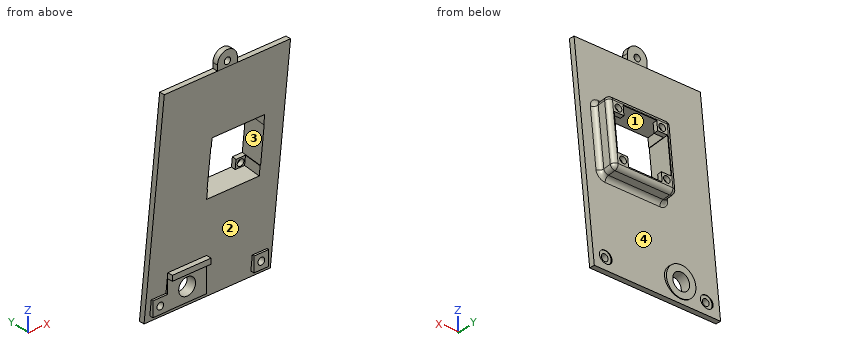
from build123d import *

# Parameters (mm, degrees)
EXTRUDE_1_DEPTH             = 60
EXTRUDE_2_REACH             = 118.966
SKETCH_3_W                  = 7
SKETCH_3_H                  = 7
SKETCH_4_R                  = 1.6
CUT_EXTRUDE_1_DEPTH         = 117.965806969
SKETCH_5_R                  = 3
CUT_EXTRUDE_2_DEPTH         = 1.2
EXTRUDE_3_REACH             = 118.966
SKETCH_6_W                  = 18.446856435
SKETCH_6_H                  = 14
SKETCH_7_W                  = 18.446856435
SKETCH_7_H                  = 2.5
EXTRUDE_4_DEPTH             = 2.5
EXTRUDE_4_DIRECTION_2_REACH = 118.966
SKETCH_8_R                  = 4
CUT_EXTRUDE_3_DEPTH         = 117.965806969
EXTRUDE_5_REACH             = 119.4
SKETCH_9_R                  = 7
SKETCH_11_R                 = 4
CUT_EXTRUDE_5_DEPTH         = 117.965806969
SKETCH_12_W                 = 30
SKETCH_12_H                 = 32
EXTRUDE_6_DEPTH             = 7.5
SKETCH_13_W                 = 25
SKETCH_13_H                 = 27
CUT_EXTRUDE_6_DEPTH         = 120.314910243
SKETCH_14_W                 = 4.5
SKETCH_14_H                 = 4.5
SKETCH_14_R                 = 1.6
EXTRUDE_7_DEPTH             = 2
FILLET_2_R                  = 2
SKETCH_15_W                 = 25.4
SKETCH_15_H                 = 18
CUT_EXTRUDE_7_DEPTH         = 120.314910243
SKETCH_16_R                 = 1.5
EXTRUDE_8_DEPTH             = 2.5


with BuildPart() as part:
    # 草图2 → 凸台-拉伸1 (new body)
    with BuildSketch(Plane(origin=(0, 0, 0), x_dir=(0, 0, -1), z_dir=(1, 0, 0))):
        Polygon((100, 28), (0, 17), (0, 14.484920478), (100, 25.484920478), align=None)
    extrude(amount=-EXTRUDE_1_DEPTH)

    # 凸台-拉伸2: up to this plane
    extrude_2_end = Plane(origin=(-60, 14.484920478, 0), z_dir=(0, -0.9940043559354329, -0.10934047915289775))
    # 草图3 → 凸台-拉伸2 (add, up to the surface)
    with BuildSketch(Plane(origin=(0, 23.484920478, 0), x_dir=(1, 0, 0), z_dir=(0, 1, 0)), mode=Mode.PRIVATE) as extrude_2_sk1:
        with Locations((-54, 94)):
            Rectangle(SKETCH_3_W, SKETCH_3_H)
    extrude_2_tool1 = split(extrude(extrude_2_sk1.sketch, amount=EXTRUDE_2_REACH, mode=Mode.PRIVATE), bisect_by=extrude_2_end, keep=Keep.BOTH, mode=Mode.PRIVATE)
    add(extrude_2_tool1.solids().sort_by_distance((-54, 23.48492, -94))[0])
    # 草图3 → 凸台-拉伸2 (add, up to the surface)
    with BuildSketch(Plane(origin=(0, 23.484920478, 0), x_dir=(1, 0, 0), z_dir=(0, 1, 0)), mode=Mode.PRIVATE) as extrude_2_sk2:
        with Locations((-6, 94)):
            Rectangle(SKETCH_3_W, SKETCH_3_H)
    extrude_2_tool2 = split(extrude(extrude_2_sk2.sketch, amount=EXTRUDE_2_REACH, mode=Mode.PRIVATE), bisect_by=extrude_2_end, keep=Keep.BOTH, mode=Mode.PRIVATE)
    add(extrude_2_tool2.solids().sort_by_distance((-6, 23.48492, -94))[0])

    # 草图4 → 切除-拉伸1 (cut, through all)
    with BuildSketch(Plane.XZ.offset(-23.484920478)):
        with Locations(Location((-54, -94, 0), (0, 0, 270))):
            Circle(SKETCH_4_R)
        with Locations(Location((-6, -94, 0), (0, 0, 90))):
            Circle(SKETCH_4_R)
    extrude(amount=-CUT_EXTRUDE_1_DEPTH, mode=Mode.SUBTRACT)

    # 草图5 → 切除-拉伸2 (cut)
    with BuildSketch(Plane(origin=(0, 28, 0), x_dir=(1, 0, 0), z_dir=(0, 1, 0))):
        with Locations(Location((-54, 94, 0), (0, 0, 270))):
            Circle(SKETCH_5_R)
        with Locations(Location((-6, 94, 0), (0, 0, 270))):
            Circle(SKETCH_5_R)
    extrude(amount=-CUT_EXTRUDE_2_DEPTH, mode=Mode.SUBTRACT)

    # 凸台-拉伸3: up to this plane
    extrude_3_end = Plane(origin=(-60, 14.484920478, 0), z_dir=(0, -0.9940043559354329, -0.10934047915289775))
    # 草图6 → 凸台-拉伸3 (add, up to the surface)
    with BuildSketch(Plane(origin=(0, 23.484920478, 0), x_dir=(1, 0, 0), z_dir=(0, 1, 0)), mode=Mode.PRIVATE) as extrude_3_sk1:
        with Locations((-41.276571782, 90.4)):
            Rectangle(SKETCH_6_W, SKETCH_6_H)
    extrude_3_tool1 = split(extrude(extrude_3_sk1.sketch, amount=EXTRUDE_3_REACH, mode=Mode.PRIVATE), bisect_by=extrude_3_end, keep=Keep.BOTH, mode=Mode.PRIVATE)
    add(extrude_3_tool1.solids().sort_by_distance((-41.276572, 23.48492, -90.4))[0])

    # 草图7 → 凸台-拉伸4 (add)
    with BuildSketch(Plane.XZ.offset(-23.484920478)):
        with Locations((-41.276571782, -82.75)):
            Rectangle(SKETCH_7_W, SKETCH_7_H)
    extrude(amount=EXTRUDE_4_DEPTH)

    # 草图7 → 凸台-拉伸4 direction 2 (add, up to next)
    with BuildSketch(Plane.XZ.offset(-23.484920478), mode=Mode.PRIVATE) as extrude_4_direction_2_sk1:
        with Locations((-41.276571782, -82.75)):
            Rectangle(SKETCH_7_W, SKETCH_7_H)
    extrude_4_direction_2_tool1 = extrude(extrude_4_direction_2_sk1.sketch, amount=-EXTRUDE_4_DIRECTION_2_REACH, mode=Mode.PRIVATE) - part.part
    add(extrude_4_direction_2_tool1.solids().sort_by_distance((-41.276572, 23.48492, -82.75))[0])

    # 草图8 → 切除-拉伸3 (cut, through all)
    with BuildSketch(Plane.XZ.offset(-23.484920478)):
        with Locations(Location((-41.276571782, -90.8, 0), (0, 0, 270))):
            Circle(SKETCH_8_R)
    extrude(amount=-CUT_EXTRUDE_3_DEPTH, mode=Mode.SUBTRACT)

    # 凸台-拉伸5: up to this plane
    extrude_5_end = Plane(origin=(-60, 28, -100), z_dir=(0, 0.9940043559354329, 0.10934047915289762))
    # 草图9 → 凸台-拉伸5 (add, up to the surface)
    with BuildSketch(Plane(origin=(0, 28, 0), x_dir=(1, 0, 0), z_dir=(0, 1, 0)), mode=Mode.PRIVATE) as extrude_5_sk1:
        with Locations(Location((-41.276571782, 90.8, 0), (0, 0, 270))):
            Circle(SKETCH_9_R)
    extrude_5_tool1 = split(extrude(extrude_5_sk1.sketch, amount=-EXTRUDE_5_REACH, mode=Mode.PRIVATE), bisect_by=extrude_5_end, keep=Keep.BOTH, mode=Mode.PRIVATE)
    add(extrude_5_tool1.solids().sort_by_distance((-41.276572, 28, -90.8))[0])

    # 草图11 → 切除-拉伸5 (cut, through all)
    with BuildSketch(Plane.XZ.offset(-23.484920478)):
        with Locations(Location((-41.276571782, -90.8, 0), (0, 0, 270))):
            Circle(SKETCH_11_R)
    extrude(amount=-CUT_EXTRUDE_5_DEPTH, mode=Mode.SUBTRACT)

    # 草图12 → 凸台-拉伸6 (add)
    with BuildSketch(Plane(origin=(0, 16.796759214, 1.847643513), x_dir=(1, 0, 0), z_dir=(0, 0.994004355935433, 0.10934047915289764))):
        with Locations((-22, 44.46196901)):
            Rectangle(SKETCH_12_W, SKETCH_12_H)
    extrude(amount=EXTRUDE_6_DEPTH)

    # 草图13 → 切除-拉伸6 (cut, through all)
    with BuildSketch(Plane(origin=(0, 24.251791883, 2.667697107), x_dir=(1, 0, 0), z_dir=(0, 0.994004355935433, 0.10934047915289753))):
        with Locations((-22, 44.46196901)):
            Rectangle(SKETCH_13_W, SKETCH_13_H)
    extrude(amount=-CUT_EXTRUDE_6_DEPTH, mode=Mode.SUBTRACT)

    # 草图14 → 凸台-拉伸7 (add)
    # profile 1 of 4: a face of its own
    with BuildSketch(Plane(origin=(0, 24.251791883, 2.667697107), x_dir=(1, 0, 0), z_dir=(0, 0.994004355935433, 0.10934047915289753))):
        with Locations((-32.25, 55.71196901)):
            Rectangle(SKETCH_14_W, SKETCH_14_H)
        with Locations(Location((-32.4, 55.86196901, 0), (0, 0, 270))):
            Circle(SKETCH_14_R, mode=Mode.SUBTRACT)
    # profile 2 of 4: a face of its own
    with BuildSketch(Plane(origin=(0, 24.251791883, 2.667697107), x_dir=(1, 0, 0), z_dir=(0, 0.994004355935433, 0.10934047915289753))):
        with Locations((-32.25, 33.21196901)):
            Rectangle(SKETCH_14_W, SKETCH_14_H)
        with Locations(Location((-32.4, 33.06196901, 0), (0, 0, 90))):
            Circle(SKETCH_14_R, mode=Mode.SUBTRACT)
    # profile 3 of 4: a face of its own
    with BuildSketch(Plane(origin=(0, 24.251791883, 2.667697107), x_dir=(1, 0, 0), z_dir=(0, 0.994004355935433, 0.10934047915289753))):
        with Locations((-11.75, 33.21196901)):
            Rectangle(SKETCH_14_W, SKETCH_14_H)
        with Locations(Location((-11.6, 33.06196901, 0), (0, 0, 270))):
            Circle(SKETCH_14_R, mode=Mode.SUBTRACT)
    # profile 4 of 4: a face of its own
    with BuildSketch(Plane(origin=(0, 24.251791883, 2.667697107), x_dir=(1, 0, 0), z_dir=(0, 0.994004355935433, 0.10934047915289753))):
        with Locations((-11.75, 55.71196901)):
            Rectangle(SKETCH_14_W, SKETCH_14_H)
        with Locations(Location((-11.6, 55.86196901, 0), (0, 0, 90))):
            Circle(SKETCH_14_R, mode=Mode.SUBTRACT)
    extrude(amount=-EXTRUDE_7_DEPTH)

    # 圆角2
    fillet_2_edges = [part.edges().sort_by_distance(p)[0] for p in [
        (-7, 21.658252209, -42.347747356),
        (-7, 23.636320877, -26.033650864),
        (-22, 23.407699876, -58.251817051),
        (-7, 27.13521621, -57.841790254),
        (-37, 21.658252209, -42.347747356),
        (-37, 27.13521621, -57.841790254),
        (-22, 19.908804543, -26.443677661),
        (-37, 23.636320877, -26.033650864),
        (-7, 29.113284879, -41.527693762),
        (-22, 30.862732545, -57.431763457),
        (-37, 29.113284879, -41.527693762),
        (-22, 27.363837212, -25.623624067),
    ]]
    fillet(fillet_2_edges, radius=FILLET_2_R)

    # 草图15 → 切除-拉伸7 (cut, through all)
    with BuildSketch(Plane(origin=(0, 24.251791883, 2.667697107), x_dir=(1, 0, 0), z_dir=(0, 0.994004355935433, 0.10934047915289753))):
        with Locations((-22, 44.46196901)):
            Rectangle(SKETCH_15_W, SKETCH_15_H)
    extrude(amount=-CUT_EXTRUDE_7_DEPTH, mode=Mode.SUBTRACT)

    # 草图16 → 凸台-拉伸8 (add)
    with BuildSketch(Plane(origin=(0, 14.484920478, 0), x_dir=(1, 0, 0), z_dir=(0, 1, 0))):
        with BuildLine():
            Line((-34.7, -2.5), (-34.7, 0))
            Line((-34.7, 0), (-25.3, 0))
            Line((-25.3, 0), (-25.3, -2.5))
            ThreePointArc((-25.3, -2.5), (-30, -7.2), (-34.7, -2.5))
        make_face()
        with Locations(Location((-30, -2.5, 0), (0, 0, 270))):
            Circle(SKETCH_16_R, mode=Mode.SUBTRACT)
    extrude(amount=EXTRUDE_8_DEPTH)


solid = part.part
Geometry: final body of the model. Coordinates: model frame, mm. Face numbers are marked on the shaded views. Give positions to 0.01 mm unless a question says otherwise; leave off trailing zeros. Loops run counter-clockwise (first coordinate to the right, second up) from the corner with the lowest first, then second, coordinate; pieces in that order, holes last. Notation, with made-up numbers: (69, 32) - (83, 32) arc R16 cw to (83, 58) - close; hole circle Ø11 at (-8, -13.75). An arc over 180 degrees is marked (long way). One line per question, with ' | ' between items. Start each with the question number.
(1) Ray query, line 1 (X direction, y = 24.4, z = -90.8); line 2 (X direction, y = 25.95, z = -94); line 3 (Z direction, x = -54, y = 27.45). Return the intervals inside material, ascending. Write a range as from..to.
(2) Contact query for flat-ended pins moving along their axis: pin 1 (5 mm diameter, centred on y = 16.5, z = -63, fed in from +X); pin 2 (0.5 mm diameter, centred on x = -5.5, y = 24.5, fed in from -Z); pin 3 (4 mm diameter, centred on x = -54, z = -94, fed in from -Y); pin 4 (2 mm diameter, centred on x = -41.5, y = 17.5, fed in from +Z). Output: stop coordinate, or through.
(3) Section query A-A on z = -82.5. Return loops of the section in (x, y) (3 decimals).
(4) Pull-direction query (Y, two-part tool) for the marked faces 1, 2, 3 and 4; classes: released by +Y, released by -Y, zero draft, split by the parting line, or undercut.
(5) Section query B-B on z = -5. Return loops of the section in (x, y), then the cut area to 3 significant figures.
The answers:
1) line 1: -57.5..-45.28, -37.28..-32.05, -9.5..-2.5 | line 2: -60..-55.6, -52.4..-43.68, -38.88..-7.6, -4.4..0 | line 3: -100..-97
2) pin 1: through | pin 2: z = -97.5 | pin 3: y = 23.48 | pin 4: z = 0
3) outline: (-60, 23.56) - (-50.5, 23.56) - (-50.5, 20.985) - (-32.053, 20.985) - (-32.053, 23.56) - (0, 23.56) - (0, 26.075) - (-60, 26.075) - close
4) face 1: undercut | face 2: released by -Y | face 3: zero draft | face 4: released by +Y
5) outline: (-60, 15.03) - (0, 15.03) - (0, 17.55) - (-60, 17.55) - close | area: 151 mm2
